from build123d import *

# Parameters (mm, degrees)
BOSS_EXTRUDE1_DEPTH = 1
FILLET2_R           = 1
SKETCH3_W           = 10
SKETCH3_H           = 7
BOSS_EXTRUDE2_DEPTH = 2
SKETCH4_W           = 22
SKETCH4_H           = 22
BOSS_EXTRUDE3_DEPTH = 2
SKETCH5_W           = 22
SKETCH5_H           = 1
BOSS_EXTRUDE4_DEPTH = 2
SKETCH6_W           = 1
SKETCH6_H           = 22
BOSS_EXTRUDE5_DEPTH = 5.1
FILLET4_R           = 1
FILLET5_R           = 0.3
SKETCH7_W           = 25
SKETCH7_H           = 22
BOSS_EXTRUDE6_DEPTH = 0.8
FILLET6_R           = 0.3
SKETCH8_W           = 10
SKETCH8_H           = 7.6
CUT_EXTRUDE1_DEPTH  = 2
SKETCH9_W           = 1
SKETCH9_H           = 22
BOSS_EXTRUDE7_DEPTH = 0.8


with BuildPart() as part:
    # Sketch2 → Boss-Extrude1 (new body)
    with BuildSketch(Plane(origin=(0, 0, 0), x_dir=(0, 1, 0), z_dir=(0, 0, 1))):
        Polygon((-7.2, 11.5), (-7.2, -11.5), (-4.8, -11.5), (-4.8, -10), (4.8, -10), (4.8, -11.5), (7.2, -11.5), (7.2, 11.5), (4.8, 11.5), (4.8, 6.5), (-4.8, 6.5), (-4.8, 11.5), align=None)
    extrude(amount=BOSS_EXTRUDE1_DEPTH)

    # Fillet2
    fillet2_edges = [part.edges().sort_by_distance(p)[0] for p in [
        (11.5, 7.2, 0.5),
        (11.5, 4.8, 0.5),
        (11.5, -4.8, 0.5),
        (11.5, -7.2, 0.5),
        (-11.5, -7.2, 0.5),
        (-11.5, -4.8, 0.5),
        (-11.5, 4.8, 0.5),
        (-11.5, 7.2, 0.5),
    ]]
    fillet(fillet2_edges, radius=FILLET2_R)

    # Sketch3 → Boss-Extrude2 (add)
    with BuildSketch(Plane.XY.offset(1)):
        with Locations((1.75, 0)):
            Rectangle(SKETCH3_W, SKETCH3_H)
    extrude(amount=BOSS_EXTRUDE2_DEPTH)

    # Sketch4 → Boss-Extrude3 (add)
    with BuildSketch(Plane.XY.offset(3)):
        with Locations((1.75, 0)):
            Rectangle(SKETCH4_W, SKETCH4_H)
    extrude(amount=BOSS_EXTRUDE3_DEPTH)

    # Sketch5 → Boss-Extrude4 (add)
    with BuildSketch(Plane.YZ.offset(12.75)):
        with Locations((0, 4.5)):
            Rectangle(SKETCH5_W, SKETCH5_H)
    extrude(amount=BOSS_EXTRUDE4_DEPTH)

    # Sketch6 → Boss-Extrude5 (add)
    with BuildSketch(Plane.XY.offset(5)):
        with Locations((14.25, 0)):
            Rectangle(SKETCH6_W, SKETCH6_H)
    extrude(amount=BOSS_EXTRUDE5_DEPTH)

    # Fillet4
    fillet4_edges = [part.edges().sort_by_distance(p)[0] for p in [
        (12.75, 0, 4),
    ]]
    fillet(fillet4_edges, radius=FILLET4_R - 0.0001)  # a hair under: the kernel refuses the full size

    # Fillet5
    fillet5_edges = [part.edges().sort_by_distance(p)[0] for p in [
        (13.75, 0, 5),
    ]]
    fillet(fillet5_edges, radius=FILLET5_R)

    # Sketch7 → Boss-Extrude6 (add)
    with BuildSketch(Plane.XY.offset(10.1)):
        with Locations((2.25, 0)):
            Rectangle(SKETCH7_W, SKETCH7_H)
    extrude(amount=BOSS_EXTRUDE6_DEPTH)

    # Fillet6
    fillet6_edges = [part.edges().sort_by_distance(p)[0] for p in [
        (13.75, 0, 10.1),
    ]]
    fillet(fillet6_edges, radius=FILLET6_R)

    # Sketch8 → Cut-Extrude1 (cut)
    with BuildSketch(Plane.XY.offset(10.9)):
        with Locations((8.75, 2.84)):
            Rectangle(SKETCH8_W, SKETCH8_H)
    extrude(amount=-CUT_EXTRUDE1_DEPTH, mode=Mode.SUBTRACT)

    # Sketch9 → Boss-Extrude7 (add)
    with BuildSketch(Plane(origin=(0, 0, 10.1), x_dir=(1, 0, 0), z_dir=(0, 0, -1))):
        with Locations((-9.75, 0)):
            Rectangle(SKETCH9_W, SKETCH9_H)
    extrude(amount=BOSS_EXTRUDE7_DEPTH)


solid = part.part
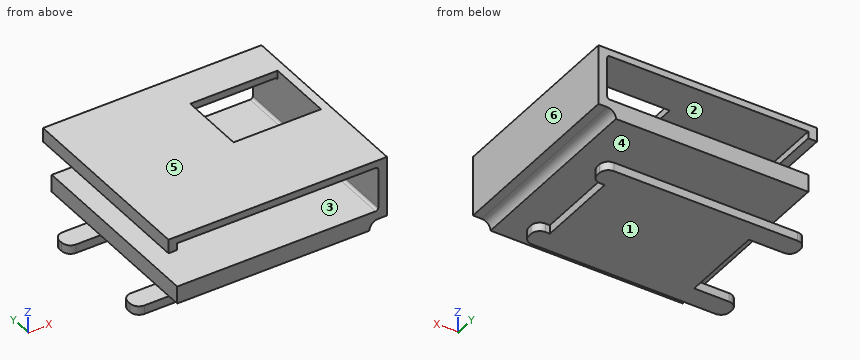
Geometry: final body of the model. Coordinates: model frame, mm. Face numbers are marked on the shaded views. A direction names the side the tool comes from. Coordinates: 2 decimals unless noted, no trailing zeros. Loops run counter-clockwise (first coordinate to the right, second up) from the corner with the lowest first, then second, coordinate; pieces in that order, holes last. Notation, with made-up numbers: (32.25, 51.5) - (66.25, 51.5) arc R12 cw to (66.25, 61.5) - close; hole circle Ø5 at (37.5, 38.25). An arc over 180 degrees is marked (long way). Put each result on its own line as item: value. Start each with the question number.
Q1. Set-up query: the marked faces 1 and 2. Return all of +Z, -Z, +X, -X, +Y, -Y with unobstructed straight access to the full face (end or side cutting, diameter ignored); none if empty.
Q2. Pin query (flat end, axial travel): pin 1 Ø0.5 at (x, y) = (14.5, -1.5) entering from -Z; pin 2 Ø0.5 at (y, z) = (0.5, 0.5) entering from +X; pin 3 Ø3 at (y, z) = (2, 4.5) entering from -X. Return the tip coordinate at first contact, or that it passes through.
Q3. Cut plane C-C, the plane x = 9.25. Return loops of the section in (y, z).
Q4. Pull-direction query (Z, two-part tool) for the marked faces 3, 4, 5 and 6; classes: released by +Z, released by -Z, zero draft, split by the parting line, or undercut.
Q5. Line query: line 1 (Z direction, x = 4, y = -5.5); line 2 (Z direction, x = -3, y = 1); line 3 (Z direction, x = 1.75, y = -9.25). Output: solid intervals per line, ascending.
Q6. Cut plane B-B, the plane x = 1.25. Return loops of the section in (y, z), and give its area (3 significant figures).
Filled sheet:
1. face 1: -Z, +X, -X, +Y, -Y
1. face 2: +Y, -Y
2. pin 1: z = 4
2. pin 2: x = 10
2. pin 3: x = -9.25
3. outline: (-11, 3) - (11, 3) - (11, 5) - (-11, 5) - close; (-11, 10.1) - (-0.96, 10.1) - (-0.96, 10.9) - (-11, 10.9) - close; (-7.2, 0) - (7.2, 0) - (7.2, 1) - (-7.2, 1) - close; (6.64, 10.1) - (11, 10.1) - (11, 10.9) - (6.64, 10.9) - close
4. face 3: undercut
4. face 4: undercut
4. face 5: released by +Z
4. face 6: zero draft
5. line 1: 0 to 1, 3 to 5, 10.1 to 10.9
5. line 2: 0 to 5, 10.1 to 10.9
5. line 3: 3 to 5, 10.1 to 10.9
6. outline: (-11, 3) - (-3.5, 3) - (-3.5, 1) - (-7.2, 1) - (-7.2, 0) - (7.2, 0) - (7.2, 1) - (3.5, 1) - (3.5, 3) - (11, 3) - (11, 5) - (-11, 5) - close; (-11, 10.1) - (11, 10.1) - (11, 10.9) - (-11, 10.9) - close
6. area: 90.0 mm²
